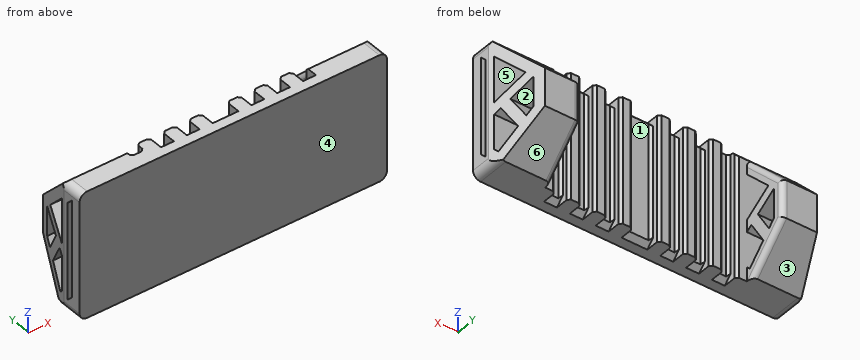
from build123d import *
from OCP.BRepFilletAPI import BRepFilletAPI_MakeChamfer

# Parameters (mm, degrees)
SKETCH1_W                 = 26
SKETCH1_H                 = 18
SKETCH1_W_2               = 134
SKETCH1_H_2               = 10
BOSS_EXTRUDE1_DEPTH       = 50
SKETCH4_W                 = 5.125
SKETCH4_H                 = 50
CUT_EXTRUDE3_DEPTH        = 4
CHAMFER1_SIZE             = 2
CHAMFER2_SIZE             = 1
CHAMFER3_SIZE             = 1
CHAMFER4_SIZE             = 1
CHAMFER5_SIZE             = 15
CHAMFER6_SIZE             = 20
CUT_EXTRUDE4_DEPTH        = 159
CHAMFER9_SIZE             = 3
CHAMFER9_SIZE2            = 2.121320344
SKETCH6_W                 = 42
SKETCH6_H                 = 2.343145751
CUT_EXTRUDE5_DEPTH        = 10
CHAMFER10_SIZE            = 3
CHAMFER10_OF_MIRROR1_SIZE = 3
CUT_EXTRUDE6_DEPTH        = 94
FILLET2_R                 = 2
BOSS_EXTRUDE2_DEPTH       = 1
SKETCH9_W                 = 4
SKETCH9_H                 = 8
CUT_EXTRUDE7_DEPTH        = 84
FILLET3_R                 = 3
FILLET4_R                 = 2


with BuildPart() as part:
    # Sketch1 → Boss-Extrude1 (new body)
    with BuildSketch(Plane.XY):
        with Locations((13, 19)):
            Rectangle(SKETCH1_W, SKETCH1_H)
        with Locations((67, 5)):
            Rectangle(SKETCH1_W_2, SKETCH1_H_2)
        with Locations((121, 19)):
            Rectangle(SKETCH1_W, SKETCH1_H)
    extrude(amount=BOSS_EXTRUDE1_DEPTH)

    # Sketch4 → Cut-Extrude3 (cut)
    with BuildSketch(Plane(origin=(0, 10, 0), x_dir=(1, 0, 0), z_dir=(0, 1, 0))):
        with Locations((33.6875, -25)):
            Rectangle(SKETCH4_W, SKETCH4_H)
        with Locations((100.3125, -25)):
            Rectangle(SKETCH4_W, SKETCH4_H)
        with Locations((43.9375, -25)):
            Rectangle(SKETCH4_W, SKETCH4_H)
        with Locations((90.0625, -25)):
            Rectangle(SKETCH4_W, SKETCH4_H)
        with Locations((54.1875, -25)):
            Rectangle(SKETCH4_W, SKETCH4_H)
        with Locations((79.8125, -25)):
            Rectangle(SKETCH4_W, SKETCH4_H)
        with Locations((64.4375, -25)):
            Rectangle(SKETCH4_W, SKETCH4_H)
        with Locations((69.5625, -25)):
            Rectangle(SKETCH4_W, SKETCH4_H)
    extrude(amount=-CUT_EXTRUDE3_DEPTH, mode=Mode.SUBTRACT)

    # Chamfer1
    chamfer1_edges = [part.edges().sort_by_distance(p)[0] for p in [
        (100.3125, 6, 50),
        (100.3125, 6, 0),
        (43.9375, 6, 0),
        (43.9375, 6, 50),
        (90.0625, 6, 50),
        (90.0625, 6, 0),
        (54.1875, 6, 0),
        (54.1875, 6, 50),
        (33.6875, 6, 0),
        (67, 6, 0),
        (67, 6, 50),
        (79.8125, 6, 50),
        (79.8125, 6, 0),
    ]]
    chamfer(chamfer1_edges, length=CHAMFER1_SIZE)

    # Chamfer2
    chamfer2_edges = [part.edges().sort_by_distance(p)[0] for p in [
        (102.875, 10, 25),
        (97.75, 10, 25),
        (41.375, 10, 25),
        (46.5, 10, 25),
        (92.625, 10, 25),
        (87.5, 10, 25),
        (51.625, 10, 25),
        (56.75, 10, 25),
        (31.125, 10, 25),
        (36.25, 10, 25),
        (61.875, 10, 25),
        (72.125, 10, 25),
        (82.375, 10, 25),
        (77.25, 10, 25),
    ]]
    chamfer(chamfer2_edges, length=CHAMFER2_SIZE)

    # Chamfer3
    chamfer3_edges = [part.edges().sort_by_distance(p)[0] for p in [
        (102.875, 6, 25),
        (97.75, 6, 25),
    ]]
    chamfer(chamfer3_edges, length=CHAMFER3_SIZE)

    # Chamfer4
    chamfer4_edges = [part.edges().sort_by_distance(p)[0] for p in [
        (41.375, 6, 25),
        (46.5, 6, 25),
        (51.625, 6, 25),
        (56.75, 6, 25),
        (61.875, 6, 25),
        (72.125, 6, 25),
        (82.375, 6, 25),
        (77.25, 6, 25),
        (92.625, 6, 25),
        (87.5, 6, 25),
        (36.25, 6, 26),
        (31.125, 6, 26),
    ]]
    chamfer(chamfer4_edges, length=CHAMFER4_SIZE)

    # Chamfer5
    chamfer5_edges = [part.edges().sort_by_distance(p)[0] for p in [
        (121, 28, 0),
        (13, 28, 0),
    ]]
    chamfer(chamfer5_edges, length=CHAMFER5_SIZE)

    # Chamfer6
    chamfer6_edges = [part.edges().sort_by_distance(p)[0] for p in [
        (13, 28, 50),
        (121, 28, 50),
    ]]
    chamfer(chamfer6_edges, length=CHAMFER6_SIZE)

    # Sketch5 → Cut-Extrude4 (cut)
    with BuildSketch(Plane(origin=(134, 0, 0), x_dir=(0, 0, -1), z_dir=(1, 0, 0))):
        Polygon((-23.118005616, 15.713850942), (-14.073840564, 21.416986315), (-16.656854249, 24), (-28.343145751, 24), align=None)
        Polygon((-24.243797472, 10), (-31.243250282, 21.099895469), (-38.343145751, 14), (-42.343145751, 10), align=None)
        Polygon((-20.98443273, 12.330381312), (-19.514923935, 10), (-2.656854249, 10), (-6.656854249, 14), (-11.173736033, 18.516881784), align=None)
    extrude(amount=-CUT_EXTRUDE4_DEPTH, mode=Mode.SUBTRACT)

    # Chamfer9: one chamfer whose edges measure the first distance from different faces: ONE call of the kernel's chamfer builder (chamfer() names one face for all edges)
    chamfer9_edges_1 = [part.edges().sort_by_distance(p)[0] for p in [
        (13, 10, 2.656854249),
    ]]
    chamfer9_side_1 = [part.faces().sort_by_distance(p)[0] for p in [
        (28.0625, 10, 0.566702358),
    ]]
    chamfer9_edges_2 = [part.edges().sort_by_distance(p)[0] for p in [
        (121, 10, 2.656854249),
    ]]
    chamfer9_side_2 = [part.faces().sort_by_distance(p)[0] for p in [
        (104.441702358, 10, 24),
    ]]
    chamfer9 = BRepFilletAPI_MakeChamfer(part.part.solid().wrapped)
    for e in chamfer9_edges_1:
        chamfer9.Add(CHAMFER9_SIZE, CHAMFER9_SIZE2, e.wrapped, chamfer9_side_1[0].wrapped)  # the first distance lies on this face
    for e in chamfer9_edges_2:
        chamfer9.Add(CHAMFER9_SIZE, CHAMFER9_SIZE2, e.wrapped, chamfer9_side_2[0].wrapped)  # the first distance lies on this face
    add(Compound.cast(chamfer9.Shape()), mode=Mode.REPLACE)

    # Sketch6 → Cut-Extrude5 (cut)
    with BuildSketch(Plane(origin=(134, 0, 0), x_dir=(0, 0, -1), z_dir=(1, 0, 0))):
        with Locations((-25, 5.171572876)):
            Rectangle(SKETCH6_W, SKETCH6_H)
    cut_extrude5 = extrude(amount=-CUT_EXTRUDE5_DEPTH, mode=Mode.SUBTRACT)

    # Chamfer10
    # the kernel refuses this chamfer: 3 mm, written as the material it adds along each edge
    with BuildSketch(Plane(origin=(134, 4, 4), x_dir=(0, -0.02749587661058634, 0.9996219169112968), z_dir=(-1, 0, 0)), Plane(origin=(134, 6.343145751, 46), x_dir=(0, 0.02749587661058648, -0.9996219169112968), z_dir=(-1, 0, 0))) as chamfer10_piece_1:
        Polygon((CHAMFER10_SIZE * 0.999621916911, CHAMFER10_SIZE * 0.0274958766106), (-CHAMFER10_SIZE * 0.0274958766106, CHAMFER10_SIZE * 0.999621916911), (0, 0), align=None)
    extrude(amount=17.715048964)

    # Mirror1: Cut-Extrude5 across plane
    add(cut_extrude5.mirror(Plane.ZY.offset(-67)), mode=Mode.SUBTRACT)

    # Chamfer10 of Mirror1
    # the kernel refuses this chamfer: 3 mm, written as the material it adds along each edge
    with BuildSketch(Plane(origin=(0, 4, 4), x_dir=(0, -0.02749587661058634, 0.9996219169112968), z_dir=(1, 0, 0)), Plane(origin=(0, 6.343145751, 46), x_dir=(0, 0.02749587661058648, -0.9996219169112968), z_dir=(1, 0, 0))) as chamfer10_of_mirror1_piece_1:
        Polygon((CHAMFER10_OF_MIRROR1_SIZE * 0.999621916911, -CHAMFER10_OF_MIRROR1_SIZE * 0.0274958766106), (-CHAMFER10_OF_MIRROR1_SIZE * 0.0274958766106, -CHAMFER10_OF_MIRROR1_SIZE * 0.999621916911), (0, 0), align=None)
    extrude(amount=17.715048964)

    # Sketch7 → Cut-Extrude6 (cut)
    with BuildSketch(Plane.XY.offset(50)):
        Polygon((0, 8), (13, 28), (0, 28), align=None)
        Polygon((121, 28), (134, 8), (134, 28), align=None)
    extrude(amount=-CUT_EXTRUDE6_DEPTH, mode=Mode.SUBTRACT)

    # Fillet2
    fillet2_edges = [part.edges().sort_by_distance(p)[0] for p in [
        (0, 4, 0),
        (134, 4, 0),
        (0, 4, 50),
        (134, 4, 50),
    ]]
    fillet(fillet2_edges, radius=FILLET2_R)

    # Sketch8 → Boss-Extrude2 (add)
    with BuildSketch(Plane(origin=(26, 0, 0), x_dir=(0, 0, -1), z_dir=(1, 0, 0))):
        Polygon((-11.173736033, 18.516881784), (-4.156854249, 11.5), (-5.656854249, 10), (0, 10), (0, 13), (-15, 28), (-30, 28), (-48, 10), (-42.343145751, 10), (-31.243250282, 21.099895469), (-24.243797472, 10), (-19.514923935, 10), (-20.98443273, 12.330381312), align=None)
        Polygon((-16.656854249, 24), (-14.073840564, 21.416986315), (-23.118005616, 15.713850942), (-28.343145751, 24), align=None, mode=Mode.SUBTRACT)
    boss_extrude2 = extrude(amount=BOSS_EXTRUDE2_DEPTH)

    # Mirror2: Boss-Extrude2 across plane
    add(boss_extrude2.mirror(Plane(origin=(67, 0, 0), x_dir=(0, 0, 1), z_dir=(1, 0, 0))))

    # Sketch9 → Cut-Extrude7 (cut)
    with BuildSketch(Plane.XY.offset(50)):
        with Locations((4, 4)):
            Rectangle(SKETCH9_W, SKETCH9_H)
        Polygon((0, 8), (0, 0), (2, 0), (2, 8), (6, 8), (6, 17.230769231), align=None)
        Polygon((13, 28), (6, 17.230769231), (6, 8), align=None)
        Polygon((121, 28), (128, 8), (128, 17.230769231), align=None)
        Polygon((132, 8), (132, 0), (134, 0), (134, 8), (128, 17.230769231), (128, 8), align=None)
        with Locations((130, 4)):
            Rectangle(SKETCH9_W, SKETCH9_H)
    extrude(amount=-CUT_EXTRUDE7_DEPTH, mode=Mode.SUBTRACT)

    # Fillet3
    fillet3_edges = [part.edges().sort_by_distance(p)[0] for p in [
        (128, 4, 0),
        (128, 4, 50),
        (6, 4, 50),
        (6, 4, 0),
    ]]
    fillet(fillet3_edges, radius=FILLET3_R)

    # Fillet4
    fillet4_edges = [part.edges().sort_by_distance(p)[0] for p in [
        (27, 20.5, 7.5),
        (27, 28, 22.5),
        (27, 19, 39),
        (107, 19, 39),
        (107, 28, 22.5),
        (107, 20.5, 7.5),
    ]]
    fillet(fillet4_edges, radius=FILLET4_R)


solid = part.part
Input: part model. Units: mm. Frame: model coordinates. Face numbers are marked on the shaded views. A direction names the side the tool comes from. Coordinates: 2 decimals unless noted, no trailing zeros. Order: outer loops, then holes, each group sorted by start corner. A loop starts at its lowest first (then second) coordinate and runs counter-clockwise, first axis right, second up.
1. Contact query for flat-ended pins moving along their axis: P1, Ø3.5, axis at x = 80, z = 18.5, coming from the +Y side (3 decimals); P2, Ø1.2, axis at y = 5.5, z = 18.5, coming from the +X side; P3, Ø4, axis at y = 6, z = 34, coming from the -X side; P4, Ø2, axis at x = 125.5, z = 34, coming from the +Y side. Output: stop coordinate, or through.
Checked values:
P1: stops at y = 6.375
P2: stops at x = 124
P3: stops at x = 6
P4: stops at y = 10
2. Cut plane A-A, the plane x = 111. Return loops of the section in (y, z), plus the area to 3 significant figures.
Checked values:
outline: (0, 0) - (13, 0) - (28, 15) - (28, 30) - (8, 50) - (0, 50) - close; hole (10, 5.66) - (11.5, 4.16) - (18.52, 11.17) - (12.33, 20.98) - (10, 19.51) - close; hole (10, 24.24) - (21.1, 31.24) - (10, 42.34) - close; hole (15.71, 23.12) - (21.42, 14.07) - (24, 16.66) - (24, 28.34) - close
area: 834 mm2
3. Draft query along Y for the marked faces 4, 5 and 6. Return one class per face: +Y half, -Y half, draft (parallel to the pull), parting line (faces both ways), or undercut.
Checked values:
face 4: -Y half
face 5: undercut
face 6: +Y half
4. Cut plane C-C, the plane y = 17.25. Count the separate pieces of the cut face and the enclosed holes in it, plus the area to 3 significant figures.
Checked values:
separate pieces: 8
enclosed holes: 0
area: 831 mm2
5. Access query for the marked faces 1, 2 and 3. Directions: +Z, -Z, +X, -X, +Y, -Y. A direction counts if a zero-diameter tool reaches every point of the face in a straight line with its end or side. Return the directions, or none.
Checked values:
face 1: +Z, -Z, +Y
face 2: +X, -X
face 3: -Z, +X, -X, +Y
6. Ray query, line 1 along Y through (x, z) = (17.5, 27); line 2 along Y through (x, z) = (59.5, 29.5); line 3 along Y through (x, z) = (64.5, 28.5). Return the intervals inside material, ascending.
Checked values:
line 1: y = 0 to 10, 14.37 to 21.87, 24 to 28
line 2: y = 0 to 10
line 3: y = 0 to 6
7. Cut plane B-B, the plane x = 67. Return loops of the section in (y, z), plus the area to 3 significant figures.
Checked values:
outline: (0, 0) - (4, 0) - (6, 2) - (6, 48) - (4, 50) - (0, 50) - close
area: 296 mm2
